Geometry: see drawing. Coordinates: mm, zero at the bounding-box minimum. Coordinates: 2 decimals unless noted, no trailing zeros. Loops run counter-clockwise (first coordinate to the right, second up) from the corner with the lowest first, then second, coordinate; pieces in that order, holes last.
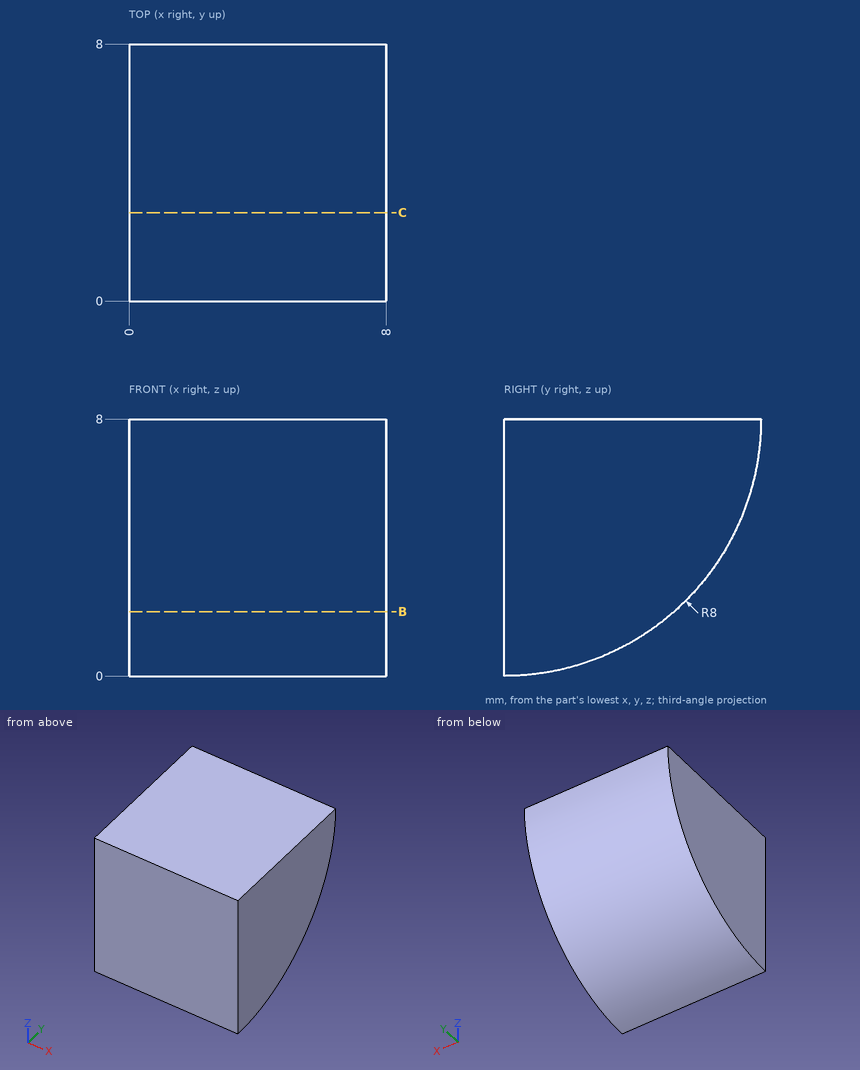
Item 1: Section query B-B (z = 2). Output: boundary loops of the cut face in (x, y).
Result:
outline: (0, 0) - (8, 0) - (8, 5.29) - (0, 5.29) - close
Item 2: Section query C-C (y = 2.75). Output: boundary loops of the cut face in (x, z), then the cut area to 3 significant figures.
Result:
outline: (0, 0.49) - (8, 0.49) - (8, 8) - (0, 8) - close
area: 60.1 mm2
Item 3: Contact query for flat-ended pins moving along their axis: P1, Ø4, axis at x = 7, y = 7, coming from the -Z side (1 decimal); P2, Ø2, axis at y = 1.5, z = 6.5, coming from the -X side; P3, Ø2, axis at x = 1, y = 5, coming from the -Z side. Output: stop coordinate, or through.
Result:
P1: stops at z = 1.8
P2: stops at x = 0
P3: stops at z = 1.07
Item 4: Line query: L1, parallel to Y at x = 4, z = 7.75; L2, parallel to Y at x = 7, z = 5.5; L3, parallel to Z at x = 1.5, y = 3.5 (1 decimal). Output: solid intervals per line, ascending.
Result:
L1: y = 0 to 8
L2: y = 0 to 7.6
L3: z = 0.8 to 8
